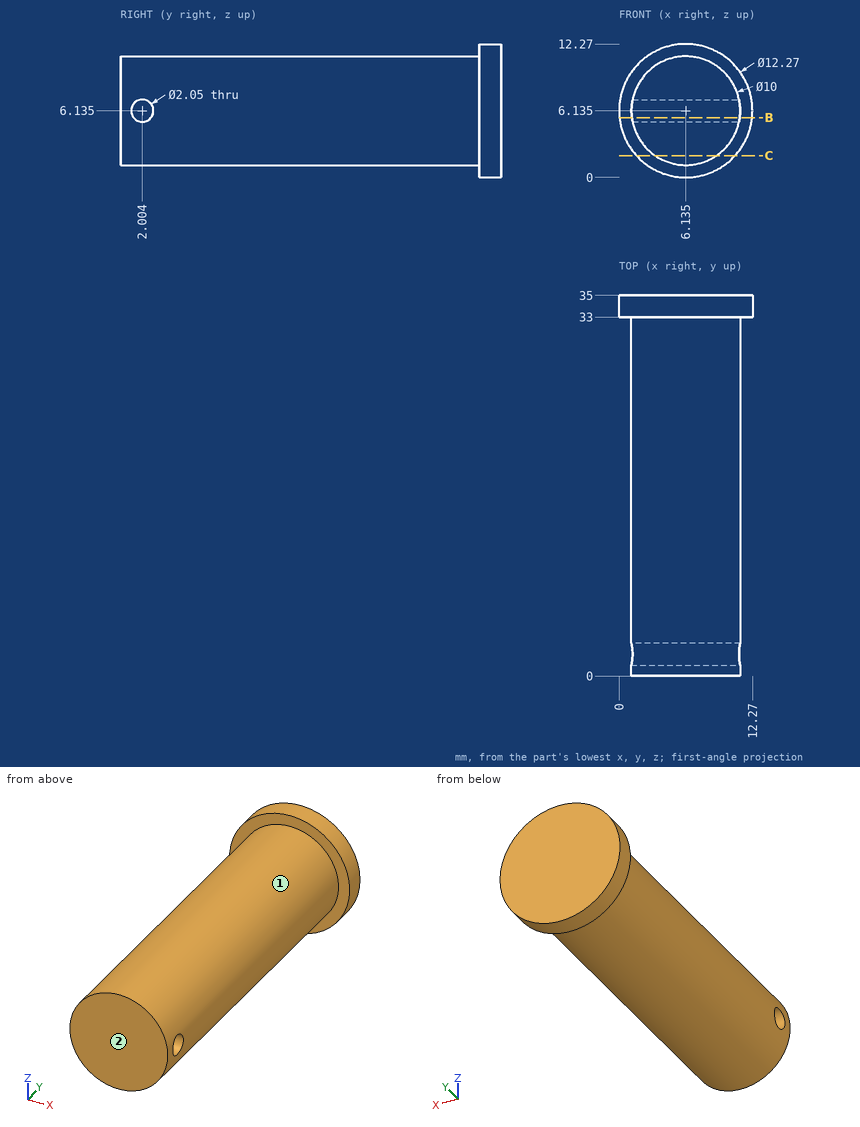
Answer from the drawing. Dimensions are ordinates in mm from the lowest x, y and z of the part. A direction names the side the tool comes from. Give positions to 0.01 mm unless a question says otherwise; leave off trailing zeros. Order: outer loops, then holes, each group sorted by start corner. A loop starts at its lowest first (then second) coordinate and runs counter-clockwise, first axis right, second up. Notation, with made-up numbers: (70, 10.5) - (89, 10.5) arc R35 cw to (89, 44.5) - close; hole circle Ø6 at (72, -5.75). An arc over 180 degrees is marked (long way). One line per item, written item: value. Start each with the question number.
1) A cutting plane is placed at B-B on z = 5.5. Give the vertices of the cut face in (x, y), then the cut area to 3 significant figures.
2) A cutting plane is placed at C-C on z = 2. Give the vertices of the cut face in (x, y).
3) Given pin 1 Ø1 at (y, z) = (14, 7) entering from +X; pin 2 Ø1 at (x, y) = (7, 15.5) entering from +Z; pin 3 Ø4 at (x, y) = (7.5, 6) entering from -Z (3 decimals), each flat-ended and moving along its own axis, determine where each tip first touches the part or whether it passes through.
4) Find the intervals of material crossed by L1, parallel to Y at x = 11.5, z = 4.5; L2, parallel to Y at x = 11, z = 5.75; L3, parallel to Y at x = 10, z = 5.5, in increasing order.
5) A tool of negligible diameter and unlimited length cuts with its end or side. For the marked faces 1 and 2, from which of +Z, -Z, +X, -X, +Y, -Y can it reach the whole face along a straight path? Write none if from no direction.
Answer sheet:
1. outline: (0.03, 33) - (1.18, 33) - (1.18, 2.81) - (11.09, 2.81) - (11.09, 33) - (12.24, 33) - (12.24, 35) - (0.03, 35) - close; (1.18, 0) - (11.09, 0) - (11.09, 1.2) - (1.18, 1.2) - close
1. area: 336 mm2
2. outline: (1.6, 33) - (3.32, 33) - (3.32, 0) - (8.95, 0) - (8.95, 33) - (10.67, 33) - (10.67, 35) - (1.6, 35) - close
3. pin 1: stops at x = 11.12
3. pin 2: stops at z = 11.12
3. pin 3: stops at z = 1.135
4. L1: y = 33 to 35
4. L2: y = 0 to 1.05, 2.95 to 35
4. L3: y = 0 to 1.2, 2.81 to 35
5. face 1: -Y
5. face 2: +Z, -Z, +X, -X, -Y
